```python
from build123d import *

# Parameters (mm, degrees)
SKETCH1_W           = 241.3
SKETCH1_H           = 266.7
BOSS_EXTRUDE1_DEPTH = 266.7
SKETCH8_W           = 228.6
SKETCH8_H           = 254
CUT_EXTRUDE4_DEPTH  = 254
SKETCH9_W           = 241.3
SKETCH9_H           = 266.7
BOSS_EXTRUDE3_DEPTH = 12.7
FILLET4_R           = 10
SKETCH10_R          = 25.4510398
CUT_EXTRUDE5_DEPTH  = 12.7
SKETCH11_R          = 12.7
CUT_EXTRUDE6_DEPTH  = 12.7


with BuildPart() as part:
    # Sketch1 → Boss-Extrude1 (new body)
    with BuildSketch(Plane(origin=(0, 0, 0), x_dir=(1, 0, 0), z_dir=(0, 1, 0))):
        Rectangle(SKETCH1_W, SKETCH1_H)
    extrude(amount=BOSS_EXTRUDE1_DEPTH)

    # Sketch8 → Cut-Extrude4 (cut)
    with BuildSketch(Plane(origin=(0, 266.7, 0), x_dir=(1, 0, 0), z_dir=(0, 1, 0))):
        Rectangle(SKETCH8_W, SKETCH8_H)
    extrude(amount=-CUT_EXTRUDE4_DEPTH, mode=Mode.SUBTRACT)

    # Sketch9 → Boss-Extrude3 (add)
    with BuildSketch(Plane(origin=(0, 266.7, 0), x_dir=(1, 0, 0), z_dir=(0, 1, 0))):
        Rectangle(SKETCH9_W, SKETCH9_H)
    extrude(amount=BOSS_EXTRUDE3_DEPTH)

    # Fillet4
    fillet4_edges = [part.edges().sort_by_distance(p)[0] for p in [
        (120.65, 279.4, 0),
        (0, 279.4, -133.35),
        (-120.65, 279.4, 0),
        (0, 279.4, 133.35),
        (0, 0, 133.35),
        (-120.65, 0, 0),
        (0, 0, -133.35),
        (120.65, 0, 0),
        (120.65, 139.7, 133.35),
        (-120.65, 139.7, 133.35),
        (-120.65, 139.7, -133.35),
        (120.65, 139.7, -133.35),
    ]]
    fillet(fillet4_edges, radius=FILLET4_R)

    # Sketch10 → Cut-Extrude5 (cut)
    with BuildSketch(Plane(origin=(120.65, 0, 0), x_dir=(0, 0, -1), z_dir=(1, 0, 0))):
        with Locations((0, 49.53971752)):
            Circle(SKETCH10_R)
    extrude(amount=-CUT_EXTRUDE5_DEPTH, mode=Mode.SUBTRACT)

    # Sketch11 → Cut-Extrude6 (cut)
    with BuildSketch(Plane(origin=(0, 279.4, 0), x_dir=(1, 0, 0), z_dir=(0, 1, 0))):
        Circle(SKETCH11_R)
    extrude(amount=-CUT_EXTRUDE6_DEPTH, mode=Mode.SUBTRACT)


solid = part.part
```
For this review, take the finished solid that the model builds, in its own axes (mm). A direction names the side the tool comes from. Coordinates: 2 decimals unless noted, no trailing zeros. Order: outer loops, then holes, each group sorted by start corner. A loop starts at its lowest first (then second) coordinate and runs counter-clockwise, first axis right, second up. Notation, with made-up numbers: (3, -13.75) -> (41, -13.75) arc R33 ccw to (41, 23.25) -> close; hole circle Ø9 at (22.25, 75). An arc over 180 degrees is marked (long way). Use CSV: the item, a comma, the result in double quotes. Start each with the question number.
Item 1: We need section C-C, the plane x = -39.5. Give the boundary of the cut face in (y, z).
Item 2: We need section A-A, the plane z = 0. Give the boundary of the cut face in (x, y).
Item 3: We need section B-B, the plane y = 114.5. Give the boundary of the cut face in (x, z).
Item 4: We need section D-D, the plane x = 0. Give the boundary of the cut face in (y, z).
Item 5: Draft analysis for pull direction Z (two halves, no side actions). For faces 4 (the face through (-2.75, 273.14, 12.4)), 5 (the face through (117.8, 137.88, -130.34)), 6 (the face through (-120.65, 138, 2)), 7 (the face through (-114.3, 141, 2)), state which applies: pulls with the +Z half, pulls with the -Z half, needs draft (parallel to the pull), parting line crosses it, or undercut.
Item 6: Wall thickness on probe 1 along X at (y, z) = (232, 39); probe 2 along Z at (x, y) = (94.5, 200); probe 3 along Y at (x, z) = (-35.5, 76): over which ranges is each line inside the solid? List them lowest first.
Item 7: For faces 1 (the face through (-117.8, 3.01, -1.73)), 2 (the face through (-2, 141, 127)), 3 (the face through (117.519, 74.774, 3.313)), list the 3-axis set-ups (+Z, -Z, +X, -X, +Y, -Y) from which the entire face can be reached by the end or side of a thin tool; tool diameter is ignored.
Derived:
1,outline,"(0, -123.35) arc R10 ccw to (10, -133.35) -> (269.4, -133.35) arc R10 ccw to (279.4, -123.35) -> (279.4, 123.35) arc R10 ccw to (269.4, 133.35) -> (10, 133.35) arc R10 ccw to (0, 123.35) -> close; hole (12.7, -127) -> (266.7, -127) -> (266.7, 127) -> (12.7, 127) -> close"
2,outline,"(-120.65, 10) arc R10 ccw to (-110.65, 0) -> (110.65, 0) arc R10 ccw to (120.65, 10) -> (120.65, 24.09) -> (114.3, 24.09) -> (114.3, 12.7) -> (-114.3, 12.7) -> (-114.3, 266.7) -> (-12.7, 266.7) -> (-12.7, 279.4) -> (-110.65, 279.4) arc R10 ccw to (-120.65, 269.4) -> close; (12.7, 266.7) -> (114.3, 266.7) -> (114.3, 74.99) -> (120.65, 74.99) -> (120.65, 269.4) arc R10 ccw to (110.65, 279.4) -> (12.7, 279.4) -> close"
3,outline,"(-120.65, -123.35) arc R10 ccw to (-110.65, -133.35) -> (110.65, -133.35) arc R10 ccw to (120.65, -123.35) -> (120.65, 123.35) arc R10 ccw to (110.65, 133.35) -> (-110.65, 133.35) arc R10 ccw to (-120.65, 123.35) -> close; hole (-114.3, -127) -> (114.3, -127) -> (114.3, 127) -> (-114.3, 127) -> close"
4,outline,"(0, -123.35) arc R10 ccw to (10, -133.35) -> (269.4, -133.35) arc R10 ccw to (279.4, -123.35) -> (279.4, -12.7) -> (266.7, -12.7) -> (266.7, -127) -> (12.7, -127) -> (12.7, 127) -> (266.7, 127) -> (266.7, 12.7) -> (279.4, 12.7) -> (279.4, 123.35) arc R10 ccw to (269.4, 133.35) -> (10, 133.35) arc R10 ccw to (0, 123.35) -> close"
5,face 4,"undercut"
5,face 5,"pulls with the -Z half"
5,face 6,"needs draft"
5,face 7,"undercut"
6,probe 1,"x = -120.65 to -114.3, 114.3 to 120.65"
6,probe 2,"z = -133.35 to -127, 127 to 133.35"
6,probe 3,"y = 0 to 12.7, 266.7 to 279.4"
7,face 1,"+Z, -Z, -X, -Y"
7,face 2,"none"
7,face 3,"+X"
